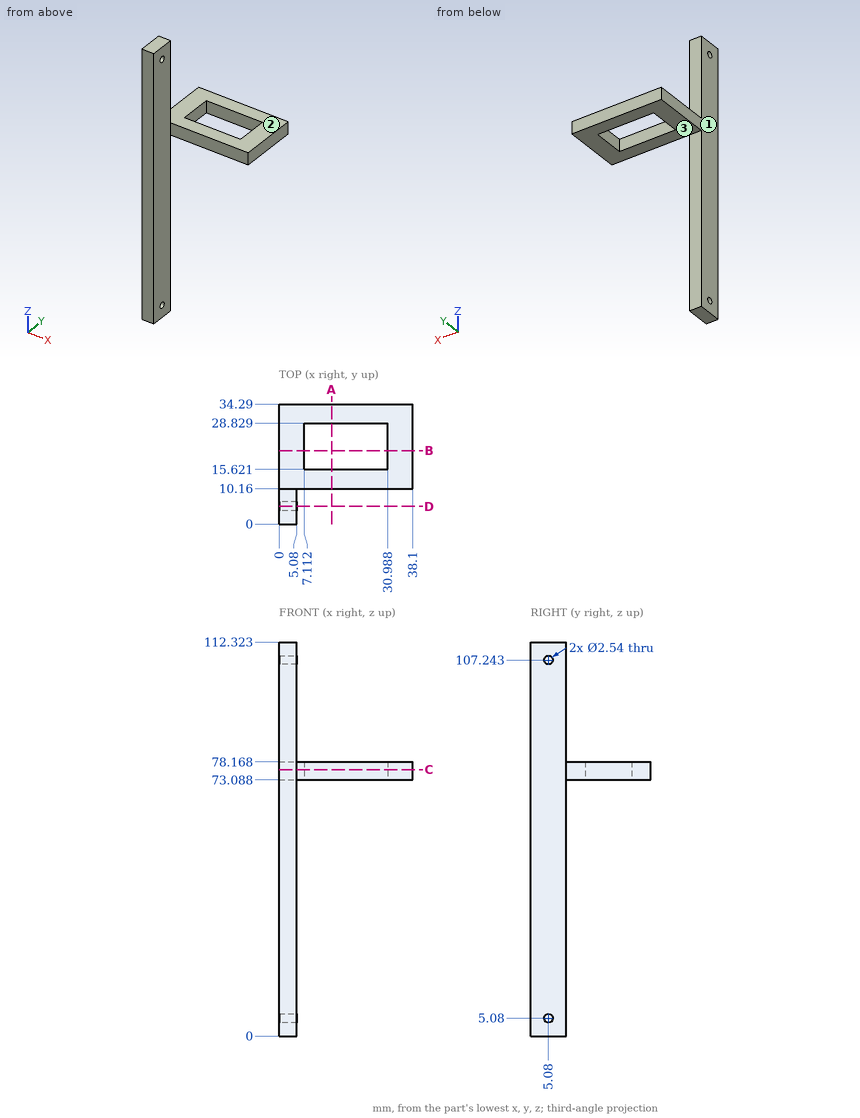
Verification items for this drawing (mm, ordinates from the low corner). A direction names the side the tool comes from. Coordinates: 2 decimals unless noted, no trailing zeros. Write each loop counter-clockwise with the first axis right and the second up, starting at its lowest first coordinate (ties: lowest second). Pieces come first, ordered by that corner, then holes. Notation, with made-up numbers: M 52,81 L 83,81 A16 ccw 83,108 Z; hole C 73.5,58 d1. An arc over 180 degrees is marked long. Answer as a JSON object with one key per item and string values. Group by question number.
(1) Cross-section at D-D, the plane y = 5.08. Record the cut outline in (x, z).
(2) Cross-section at C-C, the plane z = 76. Record the cut outline in (x, y).
(3) Cross-section at B-B, the plane y = 21. Record the cut outline in (x, z).
(4) Material ranges on line 1 (Z direction, x = 1, y = 5) (1 decimal); line 2 (Y direction, x = 1.3, z = 5.08); line 3 (Y direction, x = 2, z = 18), recorded low to high.
(5) Cross-section at A-A, the plane x = 15. Record the cut outline in (y, z).
(6) Tool access check on the marked faces 1, 2 and 3. Record the directions out of +Z, -Z, +X, -X, +Y, -Y that give a thin tool (end or side, any length) a straight path to the whole face; none if there is none.
(7) Gauge pin test, flat ends, axial feed: pin 1 (1 mm diameter, centred on x = 29, y = 15.5, fed in from -Z); pin 2 (5.5 mm diameter, centred on x = 23, z = 77, fed in from -Y); pin 3 (5.5 mm diameter, centred on x = 2, z = 89, fed in from +Y). Record the tip position at first contact, or that the pin passes through.
Reply:
{
 "1": {"outline": "M 0,0 L 5.08,0 L 5.08,3.81 L 0,3.81 Z; M 0,6.35 L 5.08,6.35 L 5.08,105.97 L 0,105.97 Z; M 0,108.51 L 5.08,108.51 L 5.08,112.32 L 0,112.32 Z"},
 "2": {"outline": "M 0,0 L 5.08,0 L 5.08,10.16 L 38.1,10.16 L 38.1,34.29 L 0,34.29 Z; hole M 7.11,15.62 L 30.99,15.62 L 30.99,28.83 L 7.11,28.83 Z"},
 "3": {"outline": "M 0,73.09 L 7.11,73.09 L 7.11,78.17 L 0,78.17 Z; M 30.99,73.09 L 38.1,73.09 L 38.1,78.17 L 30.99,78.17 Z"},
 "4": {"line 1": "0 to 3.8, 6.3 to 106, 108.5 to 112.3", "line 2": "0 to 3.81, 6.35 to 10.16", "line 3": "0 to 10.16"},
 "5": {"outline": "M 10.16,73.09 L 15.62,73.09 L 15.62,78.17 L 10.16,78.17 Z; M 28.83,73.09 L 34.29,73.09 L 34.29,78.17 L 28.83,78.17 Z"},
 "6": {"face 1": "+Z, -Z, -X, +Y, -Y", "face 2": "+Z, +X, -X, +Y", "face 3": "-Z, +X, -X, +Y"},
 "7": {"pin 1": "z = 73.09", "pin 2": "y = 10.16", "pin 3": "y = 10.16"}
}
